The model under review builds one solid part; all positions refer to its coordinate system, in mm. A direction names the side the tool comes from. Coordinates: 2 decimals unless noted, no trailing zeros. Write each loop counter-clockwise with the first axis right and the second up, starting at its lowest first coordinate (ties: lowest second). Pieces come first, ordered by that corner, then holes. Notation, with made-up numbers: (-8.5, 8) - (-2.5, 8) arc R11 ccw to (-2.5, 26) - close; hole circle Ø9 at (36, 33). An arc over 180 degrees is marked (long way). Return JSON: item names as keys, results as strings. Group by question number.
(1) Draft analysis for pull direction X (two halves, no side actions). For faces 1 (the face through (-4.044, -3.204, -1.307)), 2 (the face through (-1.555, -3.204, -4.752)), 3 (the face through (4.039, -3.204, -2.947)), 4 (the face through (-0.01, -3.2, -4.25)), state which applies: released by +X, released by -X, zero draft, split by the parting line, or undercut.
(2) Tool access review of faces 5 (the face through (4.044, -3.204, 1.307)), 6 (the face through (1.555, -3.204, 4.752)), 7 (the face through (-4.04, -3.2, 1.32)): name each direction out of +Z, -Z, +X, -X, +Y, -Y from which nothing blocks a thin tool from reaching the whole face with its end or side.
(3) For pin 1 Ø1 at (y, z) = (-4, 1.5) entering from +X; pin 2 Ø2 at (y, z) = (-3, 4) entering from -X; pin 3 Ø2 at (y, z) = (-4, -3.5) entering from -X, all flat-tipped, find the tip position at first contact; note any pin that passes through.
(4) We need section D-D on y = 1. State the section outline as (x, z) points.
(5) To check wall thickness, follow L1, parallel to Y at x = 5.25, z = 2.5; L2, parallel to Z at x = -1.25, y = -4.75; L3, parallel to Z at x = 1.5, y = -1.25. State the ranges of each line that lie inside material, in increasing order. Write a range as from..to.
(6) We need section A-A on x = 0. State the section outline as (y, z) points.
(7) We need section C-C on x = 4.5. State the section outline as (y, z) points.
(8) We need section B-B on z = 0. State the section outline as (x, y) points.
```python
from build123d import *

# Parameters (mm, degrees)
F1_DEPTH = 6.5
F0_R     = 6
F2_DEPTH = 1.5
F4_D     = 4


with BuildPart() as f1:
    # F0 (on Front) → F1 (new body)
    with BuildSketch(Plane.XZ):
        with BuildLine():
            ThreePointArc((2.938982, 3.286074), (2.498087, 3.438322), (2.217047, 3.810591))
            Line((2.217047, 3.810591), (2.04914, 4.269383))
            ThreePointArc((2.04914, 4.269383), (1.545085, 4.755283), (0.851691, 4.658458))
            Line((0.851691, 4.658458), (0.446181, 4.38598))
            ThreePointArc((0.446181, 4.38598), (0, 4.25), (-0.446181, 4.38598))
            Line((-0.446181, 4.38598), (-0.851691, 4.658458))
            ThreePointArc((-0.851691, 4.658458), (-1.545085, 4.755283), (-2.04914, 4.269383))
            Line((-2.04914, 4.269383), (-2.217047, 3.810591))
            ThreePointArc((-2.217047, 3.810591), (-2.498087, 3.438322), (-2.938982, 3.286074))
            Line((-2.938982, 3.286074), (-3.427205, 3.26816))
            ThreePointArc((-3.427205, 3.26816), (-4.045085, 2.938926), (-4.16727, 2.249549))
            Line((-4.16727, 2.249549), (-4.033437, 1.779685))
            ThreePointArc((-4.033437, 1.779685), (-4.04199, 1.313322), (-4.309192, 0.930999))
            Line((-4.309192, 0.930999), (-4.693643, 0.629537))
            ThreePointArc((-4.693643, 0.629537), (-5, 0), (-4.693643, -0.629537))
            Line((-4.693643, -0.629537), (-4.309192, -0.930999))
            ThreePointArc((-4.309192, -0.930999), (-4.04199, -1.313322), (-4.033437, -1.779685))
            Line((-4.033437, -1.779685), (-4.16727, -2.249549))
            ThreePointArc((-4.16727, -2.249549), (-4.045085, -2.938926), (-3.427205, -3.26816))
            Line((-3.427205, -3.26816), (-2.938982, -3.286074))
            ThreePointArc((-2.938982, -3.286074), (-2.498087, -3.438322), (-2.217047, -3.810591))
            Line((-2.217047, -3.810591), (-2.04914, -4.269383))
            ThreePointArc((-2.04914, -4.269383), (-1.545085, -4.755283), (-0.851691, -4.658458))
            Line((-0.851691, -4.658458), (-0.446181, -4.38598))
            ThreePointArc((-0.446181, -4.38598), (0, -4.25), (0.446181, -4.38598))
            Line((0.446181, -4.38598), (0.851691, -4.658458))
            ThreePointArc((0.851691, -4.658458), (1.545085, -4.755283), (2.04914, -4.269383))
            Line((2.04914, -4.269383), (2.217047, -3.810591))
            ThreePointArc((2.217047, -3.810591), (2.498087, -3.438322), (2.938982, -3.286074))
            Line((2.938982, -3.286074), (3.427205, -3.26816))
            ThreePointArc((3.427205, -3.26816), (4.045085, -2.938926), (4.16727, -2.249549))
            Line((4.16727, -2.249549), (4.033437, -1.779685))
            ThreePointArc((4.033437, -1.779685), (4.04199, -1.313322), (4.309192, -0.930999))
            Line((4.309192, -0.930999), (4.693643, -0.629537))
            ThreePointArc((4.693643, -0.629537), (5, 0), (4.693643, 0.629537))
            Line((4.693643, 0.629537), (4.309192, 0.930999))
            ThreePointArc((4.309192, 0.930999), (4.04199, 1.313322), (4.033437, 1.779685))
            Line((4.033437, 1.779685), (4.16727, 2.249549))
            ThreePointArc((4.16727, 2.249549), (4.045085, 2.938926), (3.427205, 3.26816))
            Line((3.427205, 3.26816), (2.938982, 3.286074))
        make_face()
    extrude(amount=F1_DEPTH)

    # F0 (on Front) → F2 (join)
    with BuildSketch(Plane.XZ):
        Circle(F0_R)
        with BuildLine():
            Line((2.04914, 4.269383), (2.217047, 3.810591))
            ThreePointArc((2.217047, 3.810591), (2.498087, 3.438322), (2.938982, 3.286074))
            Line((2.938982, 3.286074), (3.427205, 3.26816))
            ThreePointArc((3.427205, 3.26816), (4.045085, 2.938926), (4.16727, 2.249549))
            Line((4.16727, 2.249549), (4.033437, 1.779685))
            ThreePointArc((4.033437, 1.779685), (4.04199, 1.313322), (4.309192, 0.930999))
            Line((4.309192, 0.930999), (4.693643, 0.629537))
            ThreePointArc((4.693643, 0.629537), (5, 0), (4.693643, -0.629537))
            Line((4.693643, -0.629537), (4.309192, -0.930999))
            ThreePointArc((4.309192, -0.930999), (4.04199, -1.313322), (4.033437, -1.779685))
            Line((4.033437, -1.779685), (4.16727, -2.249549))
            ThreePointArc((4.16727, -2.249549), (4.045085, -2.938926), (3.427205, -3.26816))
            Line((3.427205, -3.26816), (2.938982, -3.286074))
            ThreePointArc((2.938982, -3.286074), (2.498087, -3.438322), (2.217047, -3.810591))
            Line((2.217047, -3.810591), (2.04914, -4.269383))
            ThreePointArc((2.04914, -4.269383), (1.545085, -4.755283), (0.851691, -4.658458))
            Line((0.851691, -4.658458), (0.446181, -4.38598))
            ThreePointArc((0.446181, -4.38598), (0, -4.25), (-0.446181, -4.38598))
            Line((-0.446181, -4.38598), (-0.851691, -4.658458))
            ThreePointArc((-0.851691, -4.658458), (-1.545085, -4.755283), (-2.04914, -4.269383))
            Line((-2.04914, -4.269383), (-2.217047, -3.810591))
            ThreePointArc((-2.217047, -3.810591), (-2.498087, -3.438322), (-2.938982, -3.286074))
            Line((-2.938982, -3.286074), (-3.427205, -3.26816))
            ThreePointArc((-3.427205, -3.26816), (-4.045085, -2.938926), (-4.16727, -2.249549))
            Line((-4.16727, -2.249549), (-4.033437, -1.779685))
            ThreePointArc((-4.033437, -1.779685), (-4.04199, -1.313322), (-4.309192, -0.930999))
            Line((-4.309192, -0.930999), (-4.693643, -0.629537))
            ThreePointArc((-4.693643, -0.629537), (-5, 0), (-4.693643, 0.629537))
            Line((-4.693643, 0.629537), (-4.309192, 0.930999))
            ThreePointArc((-4.309192, 0.930999), (-4.04199, 1.313322), (-4.033437, 1.779685))
            Line((-4.033437, 1.779685), (-4.16727, 2.249549))
            ThreePointArc((-4.16727, 2.249549), (-4.045085, 2.938926), (-3.427205, 3.26816))
            Line((-3.427205, 3.26816), (-2.938982, 3.286074))
            ThreePointArc((-2.938982, 3.286074), (-2.498087, 3.438322), (-2.217047, 3.810591))
            Line((-2.217047, 3.810591), (-2.04914, 4.269383))
            ThreePointArc((-2.04914, 4.269383), (-1.545085, 4.755283), (-0.851691, 4.658458))
            Line((-0.851691, 4.658458), (-0.446181, 4.38598))
            ThreePointArc((-0.446181, 4.38598), (0, 4.25), (0.446181, 4.38598))
            Line((0.446181, 4.38598), (0.851691, 4.658458))
            ThreePointArc((0.851691, 4.658458), (1.545085, 4.755283), (2.04914, 4.269383))
        make_face(mode=Mode.SUBTRACT)
        with BuildLine():
            ThreePointArc((2.938982, 3.286074), (2.498087, 3.438322), (2.217047, 3.810591))
            Line((2.217047, 3.810591), (2.04914, 4.269383))
            ThreePointArc((2.04914, 4.269383), (1.545085, 4.755283), (0.851691, 4.658458))
            Line((0.851691, 4.658458), (0.446181, 4.38598))
            ThreePointArc((0.446181, 4.38598), (0, 4.25), (-0.446181, 4.38598))
            Line((-0.446181, 4.38598), (-0.851691, 4.658458))
            ThreePointArc((-0.851691, 4.658458), (-1.545085, 4.755283), (-2.04914, 4.269383))
            Line((-2.04914, 4.269383), (-2.217047, 3.810591))
            ThreePointArc((-2.217047, 3.810591), (-2.498087, 3.438322), (-2.938982, 3.286074))
            Line((-2.938982, 3.286074), (-3.427205, 3.26816))
            ThreePointArc((-3.427205, 3.26816), (-4.045085, 2.938926), (-4.16727, 2.249549))
            Line((-4.16727, 2.249549), (-4.033437, 1.779685))
            ThreePointArc((-4.033437, 1.779685), (-4.04199, 1.313322), (-4.309192, 0.930999))
            Line((-4.309192, 0.930999), (-4.693643, 0.629537))
            ThreePointArc((-4.693643, 0.629537), (-5, 0), (-4.693643, -0.629537))
            Line((-4.693643, -0.629537), (-4.309192, -0.930999))
            ThreePointArc((-4.309192, -0.930999), (-4.04199, -1.313322), (-4.033437, -1.779685))
            Line((-4.033437, -1.779685), (-4.16727, -2.249549))
            ThreePointArc((-4.16727, -2.249549), (-4.045085, -2.938926), (-3.427205, -3.26816))
            Line((-3.427205, -3.26816), (-2.938982, -3.286074))
            ThreePointArc((-2.938982, -3.286074), (-2.498087, -3.438322), (-2.217047, -3.810591))
            Line((-2.217047, -3.810591), (-2.04914, -4.269383))
            ThreePointArc((-2.04914, -4.269383), (-1.545085, -4.755283), (-0.851691, -4.658458))
            Line((-0.851691, -4.658458), (-0.446181, -4.38598))
            ThreePointArc((-0.446181, -4.38598), (0, -4.25), (0.446181, -4.38598))
            Line((0.446181, -4.38598), (0.851691, -4.658458))
            ThreePointArc((0.851691, -4.658458), (1.545085, -4.755283), (2.04914, -4.269383))
            Line((2.04914, -4.269383), (2.217047, -3.810591))
            ThreePointArc((2.217047, -3.810591), (2.498087, -3.438322), (2.938982, -3.286074))
            Line((2.938982, -3.286074), (3.427205, -3.26816))
            ThreePointArc((3.427205, -3.26816), (4.045085, -2.938926), (4.16727, -2.249549))
            Line((4.16727, -2.249549), (4.033437, -1.779685))
            ThreePointArc((4.033437, -1.779685), (4.04199, -1.313322), (4.309192, -0.930999))
            Line((4.309192, -0.930999), (4.693643, -0.629537))
            ThreePointArc((4.693643, -0.629537), (5, 0), (4.693643, 0.629537))
            Line((4.693643, 0.629537), (4.309192, 0.930999))
            ThreePointArc((4.309192, 0.930999), (4.04199, 1.313322), (4.033437, 1.779685))
            Line((4.033437, 1.779685), (4.16727, 2.249549))
            ThreePointArc((4.16727, 2.249549), (4.045085, 2.938926), (3.427205, 3.26816))
            Line((3.427205, 3.26816), (2.938982, 3.286074))
        make_face()
    extrude(amount=-F2_DEPTH)

    # F4 (through all)
    with Locations(Plane.XZ.offset(6.5)):
        with Locations((0, 0)):
            Hole(F4_D / 2)


solid = f1.part
```
Ans:
{
 "1": {"face 1": "released by -X", "face 2": "undercut", "face 3": "released by +X", "face 4": "undercut"},
 "2": {"face 5": "+X, -Y", "face 6": "+Z, -Y", "face 7": "-X, -Y"},
 "3": {"pin 1": "x = 4.23", "pin 2": "x = -4", "pin 3": "x = -4.2"},
 "4": {"outline": "circle Ø12 at (0, 0); hole circle Ø4 at (0, 0)"},
 "5": {"L1": "0..1.5", "L2": "-4.79..-1.56, 1.56..4.79", "L3": "-4.77..-1.32, 1.32..4.77"},
 "6": {"outline": "(-6.5, -4.25) - (0, -4.25) - (0, -6) - (1.5, -6) - (1.5, -2) - (-6.5, -2) - close; (-6.5, 2) - (1.5, 2) - (1.5, 6) - (0, 6) - (0, 4.25) - (-6.5, 4.25) - close"},
 "7": {"outline": "(-6.5, -0.78) - (0, -0.78) - (0, -3.97) - (1.5, -3.97) - (1.5, 3.97) - (0, 3.97) - (0, 0.78) - (-6.5, 0.78) - close"},
 "8": {"outline": "(-6, 0) - (-5, 0) - (-5, -6.5) - (-2, -6.5) - (-2, 1.5) - (-6, 1.5) - close; (2, -6.5) - (5, -6.5) - (5, 0) - (6, 0) - (6, 1.5) - (2, 1.5) - close"}
}
